Could you check a few things on this drawing? It's one solid part, dimensions in mm from its lowest x, y, z. A direction names the side the tool comes from. Coordinates: 2 decimals unless noted, no trailing zeros. Order: outer loops, then holes, each group sorted by start corner. A loop starts at its lowest first (then second) coordinate and runs counter-clockwise, first axis right, second up. Notation, with made-up numbers: (78, -15.75) - (95, -15.75) arc R34 ccw to (95, 17.25) - close; hole circle Ø3 at (-31, -40). An arc over 180 degrees is marked (long way). Return JSON: item names as keys, results as strings. Group by question number.
1) For pin 1 Ø4.5 at (x, y) = (3.5, 2.5) entering from +Z; pin 2 Ø3 at (x, y) = (4.5, 1.5) entering from -Z; pin 3 Ø1.2 at (x, z) = (5.5, 5) entering from -Y, each with a flat end and sliding along its axis, tell me the tip position at first contact or that it passes through.
2) Imagine slicing it at C-C (x = 8.5). Write out the boundary of the cut face in (y, z), and give its area (4 significant figures).
3) Imagine slicing it at B-B (x = 5.5). Write out the boundary of the cut face in (y, z).
4) Which directions (+Z, -Z, +X, -X, +Y, -Y) give clear straight access to the entire face, cutting with the end or side of a thin tool? Please do the marked faces 1, 2 and 3.
5) Imagine slicing it at D-D (z = 4.5). Write out the boundary of the cut face in (x, y).
6) Imagine slicing it at A-A (y = 1.57). Write out the boundary of the cut face in (x, z).
7) If I drill on line 1 along Y through (x, z) = (5.2, 2.35); line 2 along Y through (x, z) = (5, 6.75); line 3 along Z through (x, y) = (7.25, 14.75), over which ranges is the centre line in solid material (lowest first)?
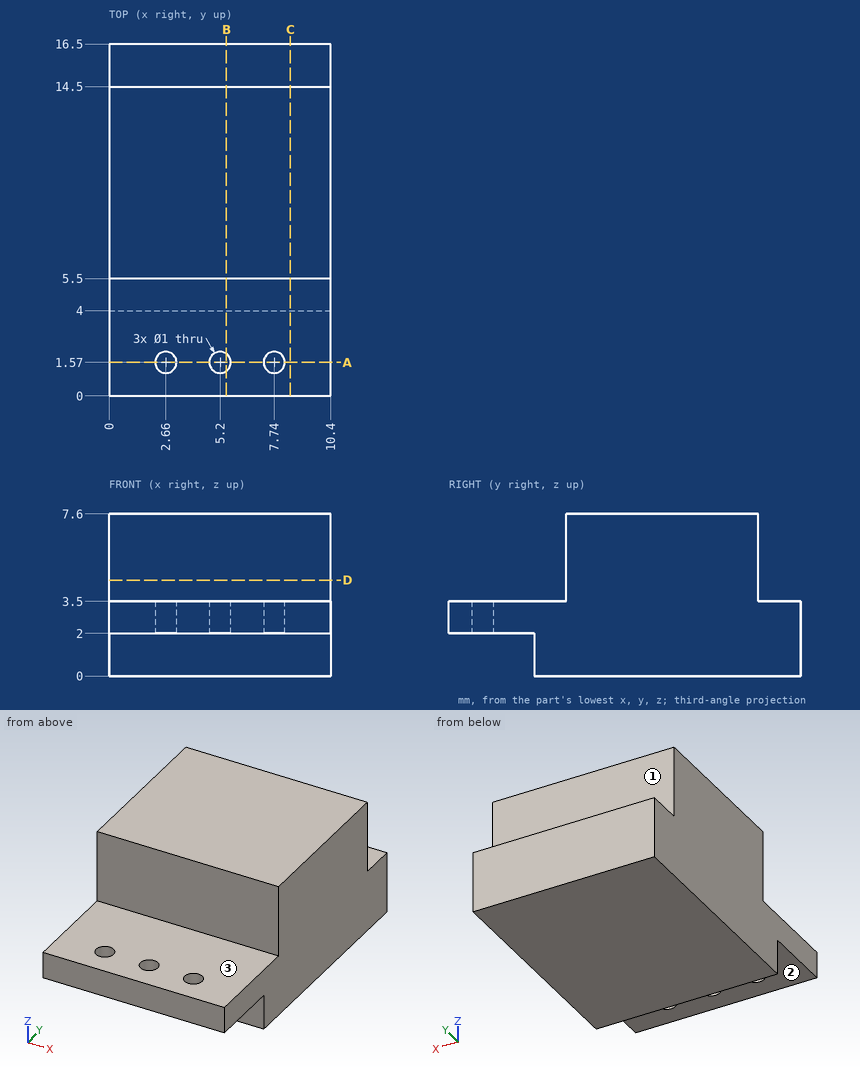
Calculated:
{
 "1": {"pin 1": "z = 3.5", "pin 2": "z = 2", "pin 3": "y = 5.5"},
 "2": {"outline": "(0, 2) - (4, 2) - (4, 0) - (16.5, 0) - (16.5, 3.5) - (14.5, 3.5) - (14.5, 7.6) - (5.5, 7.6) - (5.5, 3.5) - (0, 3.5) - close", "area": "86.65 mm2"},
 "3": {"outline": "(0, 2) - (1.17, 2) - (1.17, 3.5) - (0, 3.5) - close; (1.97, 2) - (4, 2) - (4, 0) - (16.5, 0) - (16.5, 3.5) - (14.5, 3.5) - (14.5, 7.6) - (5.5, 7.6) - (5.5, 3.5) - (1.97, 3.5) - close"},
 "4": {"face 1": "+Z, +X, -X, +Y", "face 2": "-Z, +X, -X, -Y", "face 3": "+Z, +X, -X, -Y"},
 "5": {"outline": "(0, 5.5) - (10.4, 5.5) - (10.4, 14.5) - (0, 14.5) - close"},
 "6": {"outline": "(0, 2) - (2.16, 2) - (2.16, 3.5) - (0, 3.5) - close; (3.16, 2) - (4.7, 2) - (4.7, 3.5) - (3.16, 3.5) - close; (5.7, 2) - (7.24, 2) - (7.24, 3.5) - (5.7, 3.5) - close; (8.24, 2) - (10.4, 2) - (10.4, 3.5) - (8.24, 3.5) - close"},
 "7": {"line 1": "0 to 1.07, 2.07 to 16.5", "line 2": "5.5 to 14.5", "line 3": "0 to 3.5"}
}
